Verification items for the finished model (mm, model axes). A direction names the side the tool comes from. Round coordinates to 2 decimals unless told otherwise and drop trailing zeros. Write each loop counter-clockwise with the first axis right and the second up, starting at its lowest first coordinate (ties: lowest second). Pieces come first, ordered by that corner, then holes. Notation, with made-up numbers: M 0.5,-20.75 L 10.5,-20.75 A13 cw 10.5,-15.75 Z; hole C 75.25,33.25 d10. An arc over 180 degrees is marked long. One line per question, with ' | ' between items.
from build123d import *

# Parameters (mm, degrees)
F1_DEPTH = 0.4
F5_DEPTH = 12.7
F6_DEPTH = 12.7


with BuildPart() as f1:
    # F0 (on Top) → F1 (new body)
    with BuildSketch(Plane.XY):
        Polygon((-31.5438667271, -25.7632551613), (-12.0486849532, -39.9273338113), (-19.495181774, -62.8452944863), (0, -48.6812158363), (19.495181774, -62.8452944863), (12.0486849532, -39.9273338113), (31.5438667271, -25.7632551613), (7.4464968208, -25.7632551613), (0, -2.8452944863), (-7.4464968208, -25.7632551613), align=None)
    extrude(amount=F1_DEPTH)

    # F2 (on face) → F5 (join)
    with BuildSketch(Plane.XY.offset(0.4)):
        Polygon((9.747590887, -32.8452944863), (7.4464968208, -25.7632551613), (0, -2.8452944863), (-7.4464968208, -25.7632551613), (-31.5438667271, -25.7632551613), (-12.0486849532, -39.9273338113), (-19.495181774, -62.8452944863), (0, -48.6812158363), (19.495181774, -62.8452944863), (12.0486849532, -39.9273338113), align=None)
        Polygon((31.5438667271, -25.7632551613), (9.747590887, -32.8452944863), (12.0486849532, -39.9273338113), align=None)
    extrude(amount=F5_DEPTH)

    # F6 (add): a face of the model
    f6_faces = [f1.faces().sort_by_distance(p)[0] for p in [
        (16.2459848116, -28.1239349363, 0.4),
    ]]
    extrude(f6_faces, amount=F6_DEPTH)


solid = f1.part
1. Section check C-C, the plane y = -56. Record the cut outline in (x, z).
Results:
outline: M -17.27,0 L -10.07,0 L -10.07,13.1 L -17.27,13.1 Z; M 10.07,0 L 17.27,0 L 17.27,13.1 L 10.07,13.1 Z
2. Mould release check, pull along Y, two halves, no side actions. Record for faces 4 (the face through (-21.93, -32.75, 6.46)), 5 (the face through (0, -35, 13.1)), 6 (the face through (-3.67, -14.14, 6.46)): pulls with the +Y half, pulls with the -Y half, needs draft (parallel to the pull), parting line crosses it, or undercut.
Results:
face 4: undercut | face 5: needs draft | face 6: pulls with the +Y half
3. Section check B-B, the plane z = 9. Record the cut outline in (x, y), then the cut area to 3 significant figures.
Results:
outline: M -31.54,-25.76 L -12.05,-39.93 L -19.5,-62.85 L 0,-48.68 L 19.5,-62.85 L 12.05,-39.93 L 31.54,-25.76 L 7.45,-25.76 L 0,-2.85 L -7.45,-25.76 Z | area: 1,230 mm2
4. Go/stop test with flat-tipped pins: P1, Ø3, axis at y = -55, z = 10, coming from the +X side; P2, Ø6.5, axis at x = 20, z = 9.5, coming from the +Y side; P3, Ø6, axis at y = -11, z = 10.5, coming from the +X side; P4, Ø10, axis at x = -7.5, y = -16, coming from the +Z side. Record where each tip stops, or that it passes through.
Results:
P1: stops at x = 17.43 | P2: stops at y = -25.76 | P3: stops at x = 3.62 | P4: stops at z = 13.1
5. Section check A-A, the plane x = 16.5. Record the cut outline in (y, z).
Results:
outline: M -60.67,0 L -53.63,0 L -53.63,13.1 L -60.67,13.1 Z; M -36.69,0 L -25.76,0 L -25.76,13.1 L -36.69,13.1 Z
6. Thickness scan on line 1 (X direction, y = -56.5, z = 5.25); line 2 (X direction, y = -52, z = 8); line 3 (X direction, y = -41, z = 9). Record the ranges inside material, lowest first.
Results:
line 1: x = -17.43 to -10.76, 10.76 to 17.43 | line 2: x = -15.97 to -4.57, 4.57 to 15.97 | line 3: x = -12.4 to 12.4
7. Section check D-D, the plane y = -9. Record the cut outline in (x, z), then the cut area to 3 significant figures.
Results:
outline: M -2,0 L 2,0 L 2,13.1 L -2,13.1 Z | area: 52.4 mm2
8. Tool access check on faces 1 (the face through (20, -25.763, 6)), 2 (the face through (15.824, -51.547, 6.458)), 3 (the face through (9.611, -55.664, 6.458)). Record the directions out of +Z, -Z, +X, -X, +Y, -Y that give a thin tool (end or side, any length) a straight path to the whole face; none if there is none.
Results:
face 1: +Z, -Z, +X, +Y | face 2: +Z, -Z, +X | face 3: +Z, -Z, -Y
